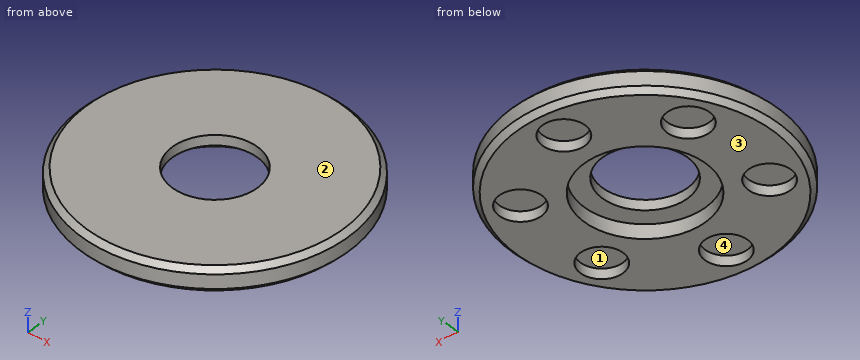
```python
from build123d import *

# Parameters (mm, degrees)
ESQUISSE1_R             = 65.794178673
BOSS_EXTRU_1_DEPTH      = 12
CONG_1_SIZE             = 2.54
ESQUISSE4_R             = 10.5
ENL_V_MAT_EXTRU_2_DEPTH = 5
ESQUISSE2_R             = 21
ENL_V_MAT_EXTRU_4_DEPTH = 94.817631043
ESQUISSE5_R             = 30
ENL_V_MAT_EXTRU_5_DEPTH = 7


with BuildPart() as part:
    # Esquisse1 → Boss.-Extru.1 (new body)
    with BuildSketch(Plane.XY):
        Circle(ESQUISSE1_R)
    extrude(amount=BOSS_EXTRU_1_DEPTH)

    # Congé1
    cong_1_edges = [part.edges().sort_by_distance(p)[0] for p in [
        (-65.794178673, 0, 0),
        (-65.794178673, 0, 12),
    ]]
    chamfer(cong_1_edges, length=CONG_1_SIZE)

    # Esquisse4 → Enlèv. mat.-Extru.2 (cut)
    with BuildSketch(Plane(origin=(0, 0, 0), x_dir=(-1, 0, 0), z_dir=(0, 0, -1))):
        with Locations((0.551144242, 48.355572121)):
            Circle(ESQUISSE4_R)
        with Locations((42.152725992, 23.700481146)):
            Circle(ESQUISSE4_R)
        with Locations((41.60158175, -24.655090975)):
            Circle(ESQUISSE4_R)
        with Locations((-0.551144242, -48.355572121)):
            Circle(ESQUISSE4_R)
        with Locations((-42.152725992, -23.700481146)):
            Circle(ESQUISSE4_R)
        with Locations((-41.60158175, 24.655090975)):
            Circle(ESQUISSE4_R)
    extrude(amount=-ENL_V_MAT_EXTRU_2_DEPTH, mode=Mode.SUBTRACT)

    # Esquisse2 → Enlèv. mat.-Extru.4 (cut, through all)
    with BuildSketch(Plane(origin=(0, 0, 0), x_dir=(-1, 0, 0), z_dir=(0, 0, -1))):
        Circle(ESQUISSE2_R)
    extrude(amount=-ENL_V_MAT_EXTRU_4_DEPTH, mode=Mode.SUBTRACT)

    # Esquisse5 → Enlèv. mat.-Extru.5 (cut)
    with BuildSketch(Plane(origin=(0, 0, 0), x_dir=(-1, 0, 0), z_dir=(0, 0, -1))):
        Circle(ESQUISSE5_R)
    extrude(amount=-ENL_V_MAT_EXTRU_5_DEPTH, mode=Mode.SUBTRACT)


solid = part.part
```
Model file for the job. Use its own axes, mm. Face numbers are marked on the shaded views. A direction names the side the tool comes from. Coordinates: 2 decimals unless noted, no trailing zeros. Write each loop counter-clockwise with the first axis right and the second up, starting at its lowest first coordinate (ties: lowest second). Pieces come first, ordered by that corner, then holes. Notation, with made-up numbers: (74.5, 59.5) - (118.5, 59.5) arc R17 cw to (118.5, 69.5) - close; hole circle Ø9 at (-6, 58). An arc over 180 degrees is marked (long way). Use a Markdown table: item, result. Add a question column.
Item 1: 3-axis set-ups, long thin cutter, end or side, ignore diameter. For the marked faces 1 and 2: which of +Z, -Z, +X, -X, +Y, -Y reach the whole face in a straight line?
Item 2: Band-saw the part on A-A, the plane y = 0. Write the cut outline in (x, z), and give its area (3 significant figures).
Item 3: Band-saw the part on B-B, the plane x = 0. Write the cut outline in (y, z).
Item 4: Drill centre lines: line 1 along Y through (x, z) = (-2.5, 2.25); line 2 along Y through (x, z) = (44.5, 1.5); line 3 along Y through (x, z) = (-8.5, 7.75). Where is each one in solid material? Low to high.
Item 5: Drop flat-ended pins along their axis: pin 1 (10.5 mm diameter, centred on x = -2.5, y = 44, fed in from -Z); pin 2 (6 mm diameter, centred on x = 30.5, z = 4, fed in from -Y); pin 3 (18 mm diameter, centred on x = 14.5, y = 1.5, fed in from -Z). Give the stop position or say it passes through.
Item 6: Two-plate mould, pull along X, no slides. Class the marked faces 3 and 4: pulls with the +X half, pulls with the -X half, needs draft (parallel to the pull), parting line crosses it, or undercut.
A:
| question | item | result |
|---|---|---|
| 1 | face 1 | -Z |
| 1 | face 2 | +Z, +X, -X, +Y, -Y |
| 2 | outline | (-65.79, 2.54) - (-63.25, 0) - (-30, 0) - (-30, 7) - (-21, 7) - (-21, 12) - (-63.25, 12) - (-65.79, 9.46) - close; (21, 7) - (30, 7) - (30, 0) - (63.25, 0) - (65.79, 2.54) - (65.79, 9.46) - (63.25, 12) - (21, 12) - close |
| 2 | area | 936 mm² |
| 3 | outline | (-65.79, 2.54) - (-63.25, 0) - (-58.84, 0) - (-58.84, 5) - (-37.87, 5) - (-37.87, 0) - (-30, 0) - (-30, 7) - (-21, 7) - (-21, 12) - (-63.25, 12) - (-65.79, 9.46) - close; (21, 7) - (30, 7) - (30, 0) - (37.87, 0) - (37.87, 5) - (58.84, 5) - (58.84, 0) - (63.25, 0) - (65.79, 2.54) - (65.79, 9.46) - (63.25, 12) - (21, 12) - close |
| 4 | line 1 | y = -65.46 to -58.4, -38.31 to -29.9, 29.9 to 38.04, 58.67 to 65.46 |
| 4 | line 2 | y = -47.04 to -33.93, -13.47 to 14.56, 34.75 to 47.04 |
| 4 | line 3 | y = -65.24 to -19.2, 19.2 to 65.24 |
| 5 | pin 1 | stops at z = 5 |
| 5 | pin 2 | stops at y = -59.77 |
| 5 | pin 3 | stops at z = 7 |
| 6 | face 3 | needs draft |
| 6 | face 4 | undercut |
